Build history of the part. All positions in model axes, mm. A direction names the side the tool comes from. Coordinates: 2 decimals unless noted, no trailing zeros. Write each loop counter-clockwise with the first axis right and the second up, starting at its lowest first coordinate (ties: lowest second). Pieces come first, ordered by that corner, then holes.
Autodesk Inventor part; units mm, degrees
ref_plane "YZ Plane" through (0, 0, 0) normal (1, 0, 0) x (0, 1, 0)
ref_plane "XZ Plane" through (0, 0, 0) normal (0, 1, 0) x (-1, 0, 0)
ref_plane "XY Plane" through (0, 0, 0) normal (0, 0, 1) x (1, 0, 0)
sketch "Sketch1" plane through (0, 0, 0) normal (0, 0, 1) x (1, 0, 0)
  circle A0 centre (0, 0) radius 2.5
  dimension "d0" = 5
extrude "Extrusion1" add sketch "Sketch1" along normal blind 50
sketch "Sketch2" plane through (0, 0, 50) normal (0, 0, 1) x (1, 0, 0)
  circle A0 centre (0, 0) radius 2.5
  circle A1 centre (0, 0) radius 1.5
  dimension "d3" = 3
extrude "Extrusion2" add sketch "Sketch2" along normal blind 5 contours A1
thread "Thread1"
sketch "Sketch3" plane through (0, 0, 0) normal (0, 0, -1) x (-1, 0, 0)
  circle A0 centre (0, 0) radius 2.5
  circle A1 centre (0, 0) radius 1.5
  dimension "d8" = 3
extrude "Extrusion3" add sketch "Sketch3" along normal blind 5 contours A1
thread "Thread2"
properties part number "spacer 5 cm"
1. Saw through at A-A on y = 0. List the corners of the cut face in (x, z), plus the area to 3 significant figures.
Computed values:
outline: (-2.5, 0) - (-1.5, 0) - (-1.5, -5) - (1.5, -5) - (1.5, 0) - (2.5, 0) - (2.5, 50) - (1.5, 50) - (1.5, 55) - (-1.5, 55) - (-1.5, 50) - (-2.5, 50) - close
area: 280 mm2
2. 3-axis set-ups, long thin cutter, end or side, ignore diameter. For faces 1 (the face through (1.5, -0.07, -2.46)), 2 (the face through (-1.5, -0.07, 52.46)), 3 (the face through (0, 0, 55)): which of +Z, -Z, +X, -X, +Y, -Y reach the whole face in a straight line?
Computed values:
face 1: -Z
face 2: +Z
face 3: +Z, +X, -X, +Y, -Y
3. Saw through at C-C on z = 29.5. List the corners of the cut face in (x, y).
Computed values:
outline: circle Ø5 at (0, 0)
4. Probe line 1 along Y through (x, z) = (-0.15, 16); line 2 along Z through (x, y) = (1.6, 0.15). List the from-to ranges inside material, lowest first.
Computed values:
line 1: y = -2.5 to 2.5
line 2: z = 0 to 50
